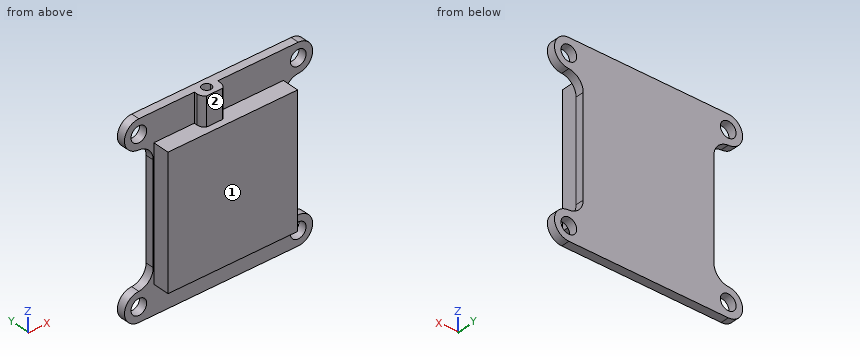
```python
from build123d import *

# Parameters (mm, degrees)
SKETCH1_R           = 1.5
BOSS_EXTRUDE1_DEPTH = 1.6
SKETCH1_3_W         = 24.8
SKETCH1_3_H         = 25
BOSS_EXTRUDE2_DEPTH = 3.2
SKETCH2_R           = 0.895817692
BOSS_EXTRUDE3_DEPTH = 5.5
CUT_EXTRUDE1_DEPTH  = 5.5


with BuildPart() as part:
    # Sketch1 → Boss-Extrude1 (new body)
    with BuildSketch(Plane(origin=(0, 0, 0), x_dir=(1, 0, 0), z_dir=(0, 1, 0))):
        with BuildLine():
            Line((-12.5, 9.510434814), (-12.5, -9.510434814))
            ThreePointArc((-12.5, -9.510434814), (-13.292059783, -11.541444415), (-15.25, -12.5))
            ThreePointArc((-15.25, -12.5), (-18, -15.25), (-15.25, -18))
            Line((-15.25, -18), (15.25, -18))
            ThreePointArc((15.25, -18), (18, -15.25), (15.25, -12.5))
            ThreePointArc((15.25, -12.5), (13.292059783, -11.541444415), (12.5, -9.510434814))
            Line((12.5, -9.510434814), (12.5, 9.510434814))
            ThreePointArc((12.5, 9.510434814), (13.292059783, 11.541444415), (15.25, 12.5))
            ThreePointArc((15.25, 12.5), (18, 15.25), (15.25, 18))
            Line((15.25, 18), (-15.25, 18))
            ThreePointArc((-15.25, 18), (-18, 15.25), (-15.25, 12.5))
            ThreePointArc((-15.25, 12.5), (-13.292059783, 11.541444415), (-12.5, 9.510434814))
        make_face()
        with Locations(Location((-15.25, -15.25, 0), (0, 0, 270))):
            Circle(SKETCH1_R, mode=Mode.SUBTRACT)
        with Locations(Location((-15.25, 15.25, 0), (0, 0, 270))):
            Circle(SKETCH1_R, mode=Mode.SUBTRACT)
        with Locations(Location((15.25, -15.25, 0), (0, 0, 270))):
            Circle(SKETCH1_R, mode=Mode.SUBTRACT)
        with Locations(Location((15.25, 15.25, 0), (0, 0, 270))):
            Circle(SKETCH1_R, mode=Mode.SUBTRACT)
    extrude(amount=BOSS_EXTRUDE1_DEPTH)

    # Sketch1<3> → Boss-Extrude2 (add)
    with BuildSketch(Plane(origin=(0, 0, 0), x_dir=(1, 0, 0), z_dir=(0, 1, 0))):
        Rectangle(SKETCH1_3_W, SKETCH1_3_H)
    extrude(amount=-BOSS_EXTRUDE2_DEPTH)

    # Sketch2 → Boss-Extrude3 (add)
    with BuildSketch(Plane.XY.offset(18)):
        with BuildLine():
            Line((-4.635, 0), (-4.1, 0))
            Line((-4.1, 0), (-4.1, 1.6))
            Line((-4.1, 1.6), (-0.7, 1.6))
            Line((-0.7, 1.6), (-0.7, 0))
            Line((-0.7, 0), (-0.165, 0))
            Line((-0.165, 0), (-0.165, -0.630150614))
            ThreePointArc((-0.165, -0.630150614), (-0.342571379, -1.352412026), (-0.834799774, -1.91))
            Line((-0.834799774, -1.91), (-3.965200226, -1.91))
            ThreePointArc((-3.965200226, -1.91), (-4.457428621, -1.352412026), (-4.635, -0.630150614))
            Line((-4.635, -0.630150614), (-4.635, 0))
        make_face()
        with Locations((-2.4, -0.15)):
            Circle(SKETCH2_R, mode=Mode.SUBTRACT)
    extrude(amount=-BOSS_EXTRUDE3_DEPTH)

    # Sketch2<2> → Cut-Extrude1 (cut)
    with BuildSketch(Plane.XY.offset(18)):
        with BuildLine():
            Line((-1.51682995, 0), (-3.28317005, 0))
            ThreePointArc((-3.28317005, 0), (-2.475266133, -1.042650182), (-1.504182308, -0.15))
            ThreePointArc((-1.504182308, -0.15), (-1.507349818, -0.074733867), (-1.51682995, 0))
        make_face()
        with BuildLine():
            ThreePointArc((-1.51682995, 0), (-2.4, 0.745817692), (-3.28317005, 0))
            Line((-3.28317005, 0), (-1.51682995, 0))
        make_face()
    extrude(amount=-CUT_EXTRUDE1_DEPTH, mode=Mode.SUBTRACT)


solid = part.part
```
Verification items for the finished model (mm, model axes). Face numbers are marked on the shaded views. A direction names the side the tool comes from. Coordinates: 2 decimals unless noted, no trailing zeros. Loops run counter-clockwise (first coordinate to the right, second up) from the corner with the lowest first, then second, coordinate; pieces in that order, holes last. Notation, with made-up numbers: (-0.5, -6.75) - (12.5, -6.75) arc R11 cw to (12.5, 8.25) - close; hole circle Ø5 at (50, 56). An arc over 180 degrees is marked (long way). Return JSON: item names as keys, results as strings.
1. Section check D-D, the plane z = -13. Record the boundary of the cut face in (x, y).
Established:
{"outline": "(-16.83, 0) - (16.83, 0) - (16.83, 1.6) - (-16.83, 1.6) - close"}
2. Section check A-A, the plane z = 15.25. Record the boundary of the cut face in (x, y) (3 decimals), then the cut area to 3 significant figures.
Established:
{"outline": "(-18, 0) - (-16.75, 0) - (-16.75, 1.6) - (-18, 1.6) - close; (-13.75, 0) - (-4.635, 0) - (-4.635, -0.63) arc R1.558 ccw to (-3.965, -1.91) - (-0.835, -1.91) arc R1.558 ccw to (-0.165, -0.63) - (-0.165, 0) - (13.75, 0) - (13.75, 1.6) - (-13.75, 1.6) - close; (16.75, 0) - (18, 0) - (18, 1.6) - (16.75, 1.6) - close; hole circle Ø1.792 at (-2.4, -0.15)", "area": "53.5 mm2"}
3. Section check C-C, the plane z = -9. Record the boundary of the cut face in (x, y), then the cut area to 3 significant figures.
Established:
{"outline": "(-12.5, 0) - (-12.4, 0) - (-12.4, -3.2) - (12.4, -3.2) - (12.4, 0) - (12.5, 0) - (12.5, 1.6) - (-12.5, 1.6) - close", "area": "119 mm2"}
4. Tool access check on the marked faces 1 and 2. Record the directions out of +Z, -Z, +X, -X, +Y, -Y that give a thin tool (end or side, any length) a straight path to the whole face; none if there is none.
Established:
{"face 1": "+Z, -Z, +X, -X, -Y", "face 2": "+Z, +X, -X, -Y"}
5. Go/stop test with flat-tipped pins: pin 1 (0.5 mm diameter, centred on y = 0.5, z = 0.5, fed in from -X); pin 2 (2 mm diameter, centred on x = -9, y = -2, fed in from -Z); pin 3 (0.5 mm diameter, centred on x = -2.5, y = 0, fed in from +Z). Record where each tip stops, or that it passes through.
Established:
{"pin 1": "stops at x = -12.5", "pin 2": "stops at z = -12.5", "pin 3": "stops at z = 12.5"}
6. Section check B-B, the plane x = 10. Record the boundary of the cut face in (y, z), then the cut area to 3 significant figures.
Established:
{"outline": "(-3.2, -12.5) - (0, -12.5) - (0, -18) - (1.6, -18) - (1.6, 18) - (0, 18) - (0, 12.5) - (-3.2, 12.5) - close", "area": "138 mm2"}
7. Thickness scan on L1, parallel to X at y = 0.9, z = -15.25; L2, parallel to X at y = 0.65, z = 15.25; L3, parallel to X at y = -1.9, z = 4. Record the ranges inside material, lowest first.
Established:
{"L1": "x = -18 to -16.75, -13.75 to 13.75, 16.75 to 18", "L2": "x = -18 to -16.75, -13.75 to -2.8, -2 to 13.75, 16.75 to 18", "L3": "x = -12.4 to 12.4"}
